from build123d import *
from OCP.BRepFilletAPI import BRepFilletAPI_MakeChamfer

# Parameters (mm, degrees)
BORE_DEPTH          = 31.494879181
BORE_DEPTH_BACK     = 31.494879181
SKETCH2_R           = 9.525
SKETCH3_W           = 1.7018
SKETCH3_H           = 4.271416332
RIDGE_DEPTH         = 31.494879181
RIDGE_PATTERN_COUNT = 18
OD_CHAMFER_SIZE     = 1.5
OD_CHAMFER_SIZE2    = 0.866025404


with BuildPart() as part:
    # Sketch1 → Bearing (revolve)
    with BuildSketch(Plane(origin=(0, 0, 0), x_dir=(0, 0, -1), z_dir=(1, 0, 0)), mode=Mode.PRIVATE) as bearing_sk:
        Polygon((-20.6375, 0), (20.6375, 0), (20.6375, -15.875), (12.7, -15.875), (12.7, -14.9479), (11.1252, -14.9479), (11.1252, -15.875), (-11.1252, -15.875), (-11.1252, -14.9479), (-12.7, -14.9479), (-12.7, -15.875), (-20.6375, -15.875), align=None)
    revolve(bearing_sk.sketch.rotate(Axis((0, 0, 20.6375), (0, 0, -1)), 270), axis=Axis((0, 0, 20.6375), (0, 0, -1)))

    # Sketch2 → Bore (cut, two sides: drawn at the far end of the back side and taken through both)
    with BuildSketch(Plane.XY.offset(-BORE_DEPTH_BACK)):
        Circle(SKETCH2_R)
    extrude(amount=BORE_DEPTH + BORE_DEPTH_BACK, mode=Mode.SUBTRACT)

    # Sketch3 → Ridge (cut, symmetric)
    with BuildSketch(Plane.XY):
        with Locations((0, 11.622625167)):
            Rectangle(SKETCH3_W, SKETCH3_H)
    ridge = extrude(amount=RIDGE_DEPTH, both=True, mode=Mode.SUBTRACT)

    # Ridge Pattern: Ridge ×18 about axis
    ridge_pattern_axis = Axis((0, 0, 0), (0, 0, 1))
    for i in range(1, RIDGE_PATTERN_COUNT):
        add(ridge.rotate(ridge_pattern_axis, i * 360 / RIDGE_PATTERN_COUNT), mode=Mode.SUBTRACT)

    # OD Chamfer: one chamfer whose edges measure the first distance from different faces: ONE call of the kernel's chamfer builder (chamfer() names one face for all edges)
    od_chamfer_edges_1 = [part.edges().sort_by_distance(p)[0] for p in [
        (-15.875, 0, 20.6375),
    ]]
    od_chamfer_side_1 = [part.faces().sort_by_distance(p)[0] for p in [
        (-15.875, 0, 16.66875),
    ]]
    od_chamfer_edges_2 = [part.edges().sort_by_distance(p)[0] for p in [
        (-15.875, 0, -20.6375),
    ]]
    od_chamfer_side_2 = [part.faces().sort_by_distance(p)[0] for p in [
        (-15.875, 0, -16.66875),
    ]]
    od_chamfer = BRepFilletAPI_MakeChamfer(part.part.solid().wrapped)
    for e in od_chamfer_edges_1:
        od_chamfer.Add(OD_CHAMFER_SIZE, OD_CHAMFER_SIZE2, e.wrapped, od_chamfer_side_1[0].wrapped)  # the first distance lies on this face
    for e in od_chamfer_edges_2:
        od_chamfer.Add(OD_CHAMFER_SIZE, OD_CHAMFER_SIZE2, e.wrapped, od_chamfer_side_2[0].wrapped)  # the first distance lies on this face
    add(Compound.cast(od_chamfer.Shape()), mode=Mode.REPLACE)


solid = part.part
The model under review builds one solid part; all positions refer to its coordinate system, in mm. Give positions to 0.01 mm unless a question says otherwise; leave off trailing zeros. Order: outer loops, then holes, each group sorted by start corner. A loop starts at its lowest first (then second) coordinate and runs counter-clockwise, first axis right, second up. Notation, with made-up numbers: (-7, 45.5) -> (47, 45.5) arc R19 cw to (47, 62.5) -> close; hole circle Ø1 at (51, 1.25). An arc over 180 degrees is marked (long way). Write item = value, one per line. Start each with the question number.
(1) Take a section at B-B (y = 0). Write out the cut boundary in (x, z) (1 decimal).
(2) For pin 1 Ø1.3 at (y, z) = (-12, -8.5) entering from -X; pin 2 Ø2 at (y, z) = (12.5, 10) entering from +X; pin 3 Ø3 at (x, z) = (7, 5) entering from -Y; pin 4 Ø10 at (x, y) = (-12.5, -12.5) entering from -Z, all flat-tipped, find the tip position at first contact; note any pin that passes through.
(3) Take a section at A-A (x = 0). Write out the cut boundary in (y, z) (1 decimal).
(4) Draft analysis for pull direction X (two halves, no side actions). For faces 1 (the cylindrical face through (6.9, 13.26, -11.9)), 2 (the flat face through (-9.61, 6.53, 0.29)), 3 (the flat face through (-11.27, 2.85, 0.29)), state which applies: +X half, -X half, draft (parallel to the pull), parting line (faces both ways), or undercut.
(5) Take a section at C-C (y = -10.5). State how many separate pieces and enclosed holes the cut face has, plus the area to 3 significant figures.
(6) For L1, parallel to X at y = 8, z = 11.5; L2, parallel to Y at x = 7, z = 18; L3, parallel to Y at x = 10, z = 0, list the stretches that pass through material, from the lowest coordinate up. Write a range as from..to.
Returned:
q1.outline = (-15.9, -19.1) -> (-15, -20.6) -> (-9.5, -20.6) -> (-9.5, 20.6) -> (-15, 20.6) -> (-15.9, 19.1) -> (-15.9, 12.7) -> (-14.9, 12.7) -> (-14.9, 11.1) -> (-15.9, 11.1) -> (-15.9, -11.1) -> (-14.9, -11.1) -> (-14.9, -12.7) -> (-15.9, -12.7) -> close; (9.5, -20.6) -> (15, -20.6) -> (15.9, -19.1) -> (15.9, -12.7) -> (14.9, -12.7) -> (14.9, -11.1) -> (15.9, -11.1) -> (15.9, 11.1) -> (14.9, 11.1) -> (14.9, 12.7) -> (15.9, 12.7) -> (15.9, 19.1) -> (15, 20.6) -> (9.5, 20.6) -> close
q2.pin_1 = -11.1
q2.pin_2 = 10.94
q2.pin_3 = -14.89
q2.pin_4 = -20.64
q3.outline = (-15.9, -19.1) -> (-15, -20.6) -> (-13.8, -20.6) -> (-13.8, 20.6) -> (-15, 20.6) -> (-15.9, 19.1) -> (-15.9, 12.7) -> (-14.9, 12.7) -> (-14.9, 11.1) -> (-15.9, 11.1) -> (-15.9, -11.1) -> (-14.9, -11.1) -> (-14.9, -12.7) -> (-15.9, -12.7) -> close; (13.8, -20.6) -> (15, -20.6) -> (15.9, -19.1) -> (15.9, -12.7) -> (14.9, -12.7) -> (14.9, -11.1) -> (15.9, -11.1) -> (15.9, 11.1) -> (14.9, 11.1) -> (14.9, 12.7) -> (15.9, 12.7) -> (15.9, 19.1) -> (15, 20.6) -> (13.8, 20.6) -> close
q4.face_1 = parting line
q4.face_2 = undercut
q4.face_3 = undercut
q5.separate_pieces = 6
q5.enclosed_holes = 0
q5.area = 653 mm²
q6.L1 = -12.63..-7.82, -5.6..-5.17, 5.17..5.6, 7.82..12.63
q6.L2 = -14.25..-9.67, -7.02..-6.46, 6.46..7.02, 9.67..14.25
q6.L3 = -12.33..-6.76, -4.79..-2.63, -0.9..0.9, 2.63..4.79, 6.76..12.33
